```python
from build123d import *

# Parameters (mm, degrees)
SKETCH2_W               = 15
SKETCH2_H               = 6.86
BOSS_EXTRUDE1_DEPTH     = 20
SKETCH4_W               = 40
SKETCH4_H               = 30
BOSS_EXTRUDE2_DEPTH     = 20
CUT_EXTRUDE_THIN1_DEPTH = 20
CUT_EXTRUDE_THIN2_DEPTH = 20
SKETCH10_W              = 15
SKETCH10_H              = 10
CUT_EXTRUDE4_DEPTH      = 20
CUT_EXTRUDE5_DEPTH      = 20


with BuildPart() as part:
    # Sketch2 → Boss-Extrude1 (new body)
    with BuildSketch(Plane.XY):
        with Locations((7.425496689, 3.579006623)):
            Rectangle(SKETCH2_W, SKETCH2_H)
    extrude(amount=BOSS_EXTRUDE1_DEPTH)

    # Sketch4 → Boss-Extrude2 (add)
    with BuildSketch(Plane.XY.offset(20)):
        with Locations((34.925496689, -7.990993377)):
            Rectangle(SKETCH4_W, SKETCH4_H)
    extrude(amount=-BOSS_EXTRUDE2_DEPTH)

    # Sketch6 → Cut-Extrude-Thin1 (cut)
    with BuildSketch(Plane.XY.offset(20)):
        Polygon((14.925491376, 0.149003146), (24.925496689, -22.915069368), (15.750749541, -26.893010391), (5.750744229, -3.828937877), align=None)
    extrude(amount=-CUT_EXTRUDE_THIN1_DEPTH, mode=Mode.SUBTRACT)

    # Sketch7 → Cut-Extrude-Thin2 (cut)
    with BuildSketch(Plane.XY.offset(20)):
        Polygon((21.92715857, 6.994080588), (32.354035132, -16.936455783), (54.974089749, -22.976067343), (57.553745552, -13.314526268), (39.594610752, -8.51939204), (31.094733139, 10.988523793), align=None)
        Polygon((22.041113505, 7.165012991), (54.974089749, 6.994080588), (54.917112281, -22.976067343), (64.917094209, -22.995078715), (64.993020621, 16.942213912), (22.09301592, 17.164878297), align=None)
    extrude(amount=-CUT_EXTRUDE_THIN2_DEPTH, mode=Mode.SUBTRACT)


with BuildPart() as body_2:
    # of the pieces the cut leaves, the one that is kept (cut_extrude_thin2_keep)
    add(part.part.solids().sort_by_distance((-0.074503311, 0.149006623, 0))[0])

    # Sketch10 → Cut-Extrude4 (cut)
    with BuildSketch(Plane(origin=(0, 7.009006623, 0), x_dir=(1, 0, 0), z_dir=(0, 1, 0))):
        with Locations((7.425496689, -10)):
            Rectangle(SKETCH10_W, SKETCH10_H)
    extrude(amount=-CUT_EXTRUDE4_DEPTH, mode=Mode.SUBTRACT)

    # Sketch11 → Cut-Extrude5 (cut)
    with BuildSketch(Plane.XY.offset(20)):
        with BuildLine():
            ThreePointArc((6.325496689, 3.60059408), (4.314702178, 5.60056495), (2.32561321, 3.579005373))
            Line((2.32561321, 3.579005373), (6.325380145, 3.579003291))
            ThreePointArc((6.325380145, 3.579003291), (6.325467553, 3.589798528), (6.325496689, 3.60059408))
        make_face()
        with BuildLine():
            Line((6.325380145, 3.579003291), (2.32561321, 3.579005373))
            ThreePointArc((2.32561321, 3.579005373), (4.325495648, 1.60059408), (6.325380145, 3.579003291))
        make_face()
        with BuildLine():
            ThreePointArc((12.92549092, 3.578999855), (10.92549773, 5.574196049), (8.925502463, 3.579001937))
            Line((8.925502463, 3.579001937), (12.92549092, 3.578999855))
        make_face()
        with BuildLine():
            Line((12.92549092, 3.578999855), (8.925502463, 3.579001937))
            ThreePointArc((8.925502463, 3.579001937), (10.923093743, 1.574197492), (12.925496689, 3.574196049))
            ThreePointArc((12.925496689, 3.574196049), (12.925495246, 3.576597954), (12.92549092, 3.578999855))
        make_face()
    extrude(amount=-CUT_EXTRUDE5_DEPTH, mode=Mode.SUBTRACT)


solid = body_2.part
```
Here's how the part is built. I have some questions about the finished solid (model axes, mm). A direction names the side the tool comes from. Coordinates: 2 decimals unless noted, no trailing zeros. Write each loop counter-clockwise with the first axis right and the second up, starting at its lowest first coordinate (ties: lowest second). Pieces come first, ordered by that corner, then holes. Notation, with made-up numbers: M 38.5,12.25 L 97.5,12.25 A26 ccw 97.5,32.25 Z; hole C 28.5,-21 d2. An arc over 180 degrees is marked long. Answer as CSV lines item,"result". Start each with the question number.
Q1. Suppose I cut it at B-B, the plane x = 11. List the corners of the cut face in (y, z) for me.
Q2. Suppose I cut it at D-D, the plane y = -0.5. List the corners of the cut face in (x, z) for me.
Q3. If we mould it in two halves opening along Z, with no side actions, what happens to faces 4 (the flat face through (7, 4, 15)), 5 (the flat face through (-0.075, 4, 2)), 6 (the flat face through (23, -8, 0))? For each: pulls with the +Z half, pulls with the -Z half, needs draft (parallel to the pull), parting line crosses it, or undercut.
Q4. Suppose I cut it at A-A, the plane z = 17.5. State how many separate pieces and enclosed holes the cut face has, then the cut area to 3 significant figures.
Q5. For faces 1 (the flat face through (40, -22.991, 10)), 2 (the flat face through (7, 0.149, 17)), 3 (the flat face through (7, 4, 5)), which set-ups out of +Z, -Z, +X, -X, +Y, -Y let a thin tool reach every point of the face, with its end or its side?
Q6. Will these pins go through, and if not, where does the flat tip stop? pin 1 Ø1 at (y, z) = (4, 10.5) entering from +X; pin 2 Ø3.5 at (y, z) = (2.5, 12) entering from -X; pin 3 Ø5.5 at (x, z) = (11, 1.5) entering from -Y; pin 4 Ø5.5 at (x, y) = (5, 5) entering from +Z.
Q7. I need wall thicknesses on probe 1 along X at (y, z) = (0.5, 10.5); probe 2 along Y at (x, z) = (2, 1.25); probe 3 along X at (y, z) = (-12, 17). Which ranges of each line are inside material? Lowest first, please. Write a range as [from, to].
Entries:
1,outline,"M 0.15,0 L 1.58,0 L 1.58,5 L 0.15,5 Z; M 0.15,15 L 1.58,15 L 1.58,20 L 0.15,20 Z; M 5.57,0 L 7.01,0 L 7.01,5 L 5.57,5 Z; M 5.57,15 L 7.01,15 L 7.01,20 L 5.57,20 Z"
2,outline,"M 15.21,0 L 25.19,0 L 25.19,20 L 15.21,20 Z"
3,face 4,"undercut"
3,face 5,"needs draft"
3,face 6,"pulls with the -Z half"
4,separate pieces,"1"
4,enclosed holes,"2"
4,area,"428 mm²"
5,face 1,"+Z, -Z, +X, -X, -Y"
5,face 2,"+Z, -Z, -X, -Y"
5,face 3,"-X, +Y, -Y"
6,pin 1,"stops at x = 23.45"
6,pin 2,"stops at x = 14.93"
6,pin 3,"stops at y = 0.15"
6,pin 4,"stops at z = 20"
7,probe 1,"x = [14.93, 24.76]"
7,probe 2,"y = [0.15, 7.01]"
7,probe 3,"x = [20.19, 30.2]"
